Design review of the part built by this model. Coordinates are the model's own, in mm. Face numbers are marked on the shaded views. Round coordinates to 2 decimals unless told otherwise and drop trailing zeros. Loops run counter-clockwise (first coordinate to the right, second up) from the corner with the lowest first, then second, coordinate; pieces in that order, holes last. Notation, with made-up numbers: M 87,3 L 92,3 A22 cw 92,17 Z; hole C 84,67.25 d6. An arc over 180 degrees is marked long. One line per item, written item: value. Start each with the question number.
Item 1: Mouldability with a two-part tool opening along X and no side actions: class the marked faces 1, 2, 3 and 4 as released by +X, released by -X, zero draft, split by the parting line, or undercut.
Item 2: We need section C-C (x = 7.5). Write out the cut boundary in (y, z).
Item 3: We need section A-A (z = 10). Write out the cut boundary in (x, y).
Item 4: We need section B-B (y = 13). Write out the cut boundary in (x, z).
Item 5: We need section D-D (y = 22.75). Write out the cut boundary in (x, z), then the cut area to 3 significant figures.
Item 6: For line 1 along Z through (x, y) = (7.5, 6); line 2 along X through (y, z) = (4.75, 10); line 3 along Y through (x, z) = (11.75, 10), list the stretches that pass through material, from the lowest coordinate up.
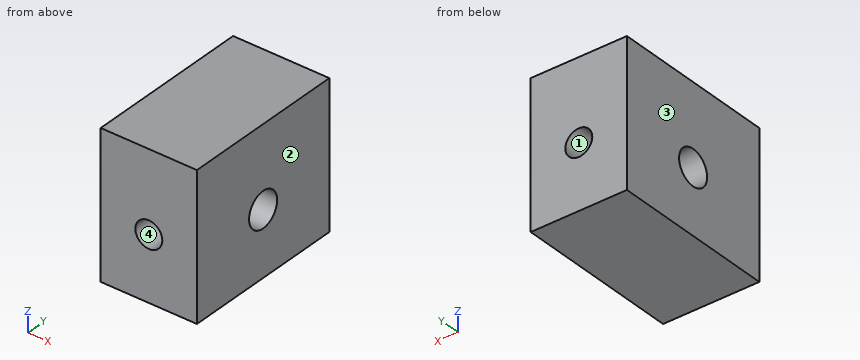
from build123d import *

# Parameters (mm, degrees)
F0_W     = 15
F0_H     = 26
F1_DEPTH = 22.5298
F3_D     = 4.2
F5_D     = 5.5


with BuildPart() as f1:
    # F0 (on Top) → F1 (new body)
    with BuildSketch(Plane.XY):
        with Locations((7.5, 13)):
            Rectangle(F0_W, F0_H)
    extrude(amount=F1_DEPTH)

    # F3 (through all)
    with Locations(Plane.XZ):
        with Locations((7.5, 10)):
            Hole(F3_D / 2)

    # F5 (through all)
    with Locations(Plane.YZ.offset(15)):
        with Locations((13, 10)):
            Hole(F5_D / 2)


solid = f1.part
A:
1. face 1: undercut
1. face 2: released by +X
1. face 3: released by -X
1. face 4: undercut
2. outline: M 0,0 L 26,0 L 26,7.9 L 14.78,7.9 A2.75 cw 11.22,7.9 L 0,7.9 Z; M 0,12.1 L 11.22,12.1 A2.75 cw 14.78,12.1 L 26,12.1 L 26,22.53 L 0,22.53 Z
3. outline: M 0,0 L 5.4,0 L 5.4,10.25 L 0,10.25 Z; M 0,15.75 L 5.4,15.75 L 5.4,26 L 0,26 Z; M 9.6,0 L 15,0 L 15,10.25 L 9.6,10.25 Z; M 9.6,15.75 L 15,15.75 L 15,26 L 9.6,26 Z
4. outline: M 0,0 L 15,0 L 15,7.25 L 0,7.25 Z; M 0,12.75 L 15,12.75 L 15,22.53 L 0,22.53 Z
5. outline: M 0,0 L 15,0 L 15,22.53 L 0,22.53 Z; hole C 7.5,10 d4.2
5. area: 324 mm2
6. line 1: 0 to 7.9, 12.1 to 22.53
6. line 2: 0 to 5.4, 9.6 to 15
6. line 3: 0 to 10.25, 15.75 to 26
